The listing builds one solid part. Answer for the finished solid, in the listing's coordinates (mm). A direction names the side the tool comes from. Give positions to 0.01 mm unless a question says otherwise; leave off trailing zeros. Order: outer loops, then holes, each group sorted by start corner. A loop starts at its lowest first (then second) coordinate and runs counter-clockwise, first axis right, second up. Notation, with made-up numbers: (-22, 19.25) - (15, 19.25) arc R23 ccw to (15, 32.25) - close; hole circle Ø9 at (-3.75, 23.25). An arc over 180 degrees is marked (long way). Answer as a JSON object with one key per item and string values. Group by question number.
Q1. Consider line 1 (Z direction, x = -13.5, y = -10); line 2 (Y direction, x = 5.5, z = 4.5); line 3 (X direction, y = -14.5, z = 1). Determine where each line is inside the solid, lowest interval first.
Q2. A cutting plane is placed at C-C, the plane z = 1. Give the vertices of the cut face in (x, y).
Q3. For faces 5 (the face through (15.14, 4.77, 10.98)), 6 (the face through (-1.669, -7.517, 2.712)), 7 (the face through (15.274, 14.968, 1.521)), determine the directions among +Z, -Z, +X, -X, +Y, -Y from which every point of the face is accessible in a straight line to the end or side of a thin tool.
Q4. A cutting plane is placed at D-D, the plane z = 4.75. Give the vertices of the cut face in (x, y) (3 decimals).
Q5. Given pin 1 (15 mm diameter, centred on x = 0, y = 0, fed in from -Z); pin 2 (7.5 mm diameter, centred on x = -0.5, y = 2, fed in from +Z); pin 3 (3 mm diameter, centred on x = 12, z = 5, fed in from -Y), each flat-ended and moving along its own axis, determine where each tip first touches the part or whether it passes through.
Q6. The mould has two halves that part along X. Classify faces 1 (the face through (-5.3, -15.5, 3)), 2 (the face through (-13.607, 15.575, 1.521)), 3 (the face through (17.5, 0, 1)), 4 (the face through (0, 6, 7.5)): released by +X, released by -X, zero draft, split by the parting line, or undercut.
from build123d import *

# Parameters (mm, degrees)
F2_W      = 35
F2_H      = 35
F2_R      = 15.875
F2_R_2    = 7.7
F3_DEPTH  = 3
F4_D      = 3.3
F4_DEPTH  = 13.905
F4_TIP    = 0.9914200214
F5_R      = 15.875
F5_R_2    = 7.7
F6_DEPTH  = 9.5
F10_R     = 7.7
F10_R_2   = 5.7
F11_DEPTH = 2
F12_SIZE  = 1.99999


# Not quite as in the source:
# - a fillet or chamfer is up to 0.001 mm smaller than in the source, because OpenCascade refuses the exact size


with BuildPart() as f3:
    # F2 (on Top) → F3 (new body)
    with BuildSketch(Plane.XY):
        Rectangle(F2_W, F2_H)
        Circle(F2_R, mode=Mode.SUBTRACT)
        Circle(F2_R)
        Circle(F2_R_2, mode=Mode.SUBTRACT)
    extrude(amount=F3_DEPTH)

    # F4
    with Locations(Plane(origin=(0, 0, 0), x_dir=(1, 0, 0), z_dir=(0, 0, -1))):
        with Locations((-13.9644660941, 13.9644660941), (-13.9644660941, -13.9644660941), (13.9644660941, -13.9644660941), (13.9644660941, 13.9644660941)):
            Hole(F4_D / 2, depth=F4_DEPTH)
            with Locations((0, 0, -(F4_DEPTH + F4_TIP / 2))):  # 118° drill point
                Cone(0, F4_D / 2, F4_TIP, mode=Mode.SUBTRACT)

    # F5 (on face) → F6 (join)
    with BuildSketch(Plane.XY.offset(3)):
        Circle(F5_R)
        Circle(F5_R_2, mode=Mode.SUBTRACT)
    extrude(amount=F6_DEPTH)

    # F7 (on Right) → F8 (revolve, cut)
    with BuildSketch(Plane.YZ):
        with BuildLine():
            ThreePointArc((-15.875, 6), (-14.8432458366, 7.75), (-15.875, 9.5))
            Line((-15.875, 9.5), (-15.875, 6))
        make_face()
    revolve(axis=Axis((0, 0, 3), (0, 0, -1)), mode=Mode.SUBTRACT)

    # F10 (on offset) → F11 (join)
    with BuildSketch(Plane.XY.offset(5.5)):
        Circle(F10_R)
        Circle(F10_R_2, mode=Mode.SUBTRACT)
    extrude(amount=F11_DEPTH)

    # F12 (size 2 in the source; OpenCascade refuses exactly that, so slightly less here)
    f12_edges = [f3.edges().sort_by_distance(p)[0] for p in [
        (-5.7, 0, 5.5),
    ]]
    chamfer(f12_edges, length=F12_SIZE)


solid = f3.part
Reply:
{
 "1": {"line 1": "z = 0 to 3", "line 2": "y = -14.89 to -5.39, 5.39 to 14.89", "line 3": "x = -17.5 to -15.53, -12.4 to 12.4, 15.53 to 17.5"},
 "2": {"outline": "(-17.5, -17.5) - (17.5, -17.5) - (17.5, 17.5) - (-17.5, 17.5) - close; hole circle Ø3.3 at (-13.96, -13.96); hole circle Ø3.3 at (-13.96, 13.96); hole circle Ø15.4 at (0, 0); hole circle Ø3.3 at (13.96, -13.96); hole circle Ø3.3 at (13.96, 13.96)"},
 "3": {"face 5": "+Z", "face 6": "-Z", "face 7": "+Z, -Z"},
 "4": {"outline": "circle Ø31.75 at (0, 0); hole circle Ø15.4 at (0, 0)"},
 "5": {"pin 1": "stops at z = 5.7", "pin 2": "stops at z = 7.5", "pin 3": "stops at y = -11.91"},
 "6": {"face 1": "zero draft", "face 2": "undercut", "face 3": "released by +X", "face 4": "undercut"}
}
